Geometry check sheet. Reference: the model listing, model coordinates, mm. Face numbers are marked on the shaded views. Coordinates: 2 decimals unless noted, no trailing zeros. Write each loop counter-clockwise with the first axis right and the second up, starting at its lowest first coordinate (ties: lowest second). Pieces come first, ordered by that corner, then holes. Notation, with made-up numbers: (44, -19) -> (85, -19) arc R21 cw to (85, -11) -> close; hole circle Ø9 at (66.5, 34). An arc over 180 degrees is marked (long way). Answer in a Markdown table with one row per item. Add a question column.
1. Cross-section at B-B on y = -7.5. Record the cut outline in (x, z), and give its area (3 significant figures).
2. Depth check by flat-ended pin: P1, Ø1.5, axis at x = 27.5, y = 3, coming from the +Z side; P2, Ø5, axis at x = 50.5, z = -10.5, coming from the +Y side; P3, Ø4, axis at x = 23, y = 2.5, coming from the +Z side. Enter the tip coordinate at first touch or a pass-through.
3. Cross-section at A-A on x = 14. Record the cut outline in (y, z).
4. Mould release check, pull along Y, two halves, no side actions. Record for the marked faces 1, 2 and 3: pulls with the +Y half, pulls with the -Y half, needs draft (parallel to the pull), parting line crosses it, or undercut.
5. Scan lines: L1, parallel to Z at x = 18, y = -2; L2, parallel to Z at x = 59.5, y = -8.5; L3, parallel to X at y = 13, z = -13.5. Record each from-to range of solid material in increasing order. Write a range as from..to.
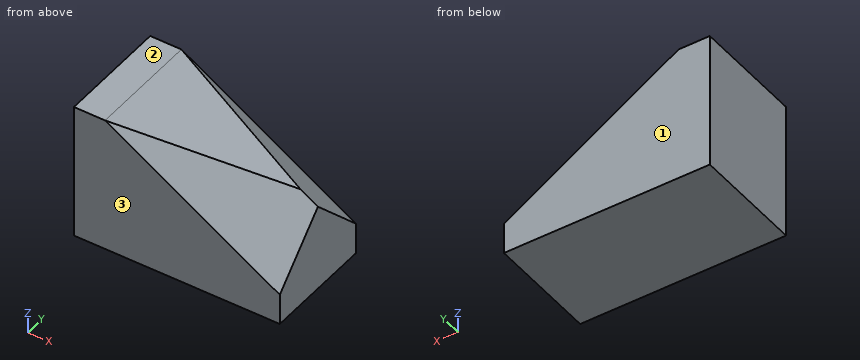
Autodesk Inventor part; units mm, degrees
ref_plane "工作平面1" through (10, 18, 0) normal (-0.3945, -0.6498, -0.6498) x (0.8548, 0, -0.519)
ref_plane "YZ Plane" through (0, 0, 0) normal (1, 0, 0) x (0, 1, 0)
ref_plane "XZ Plane" through (0, 0, 0) normal (0, 1, 0) x (-1, 0, 0)
sketch "草圖1" plane through (0, 0, 0) normal (0, 1, 0) x (-1, 0, 0)
  line L0 (0, 0) -> (-66, 0)
  line L1 (-66, 0) -> (-66, -44)
  line L2 (-66, -44) -> (0, -44)
  line L3 (0, -44) -> (0, 0)
  dimension "d0" = 66
  dimension "d1" = 44
extrude "擠出1" add sketch "草圖1" along normal mid plane 36
sketch "草圖2" plane through (0, 18, 0) normal (0, 1, 0) x (1, 0, 0)
  line L0 (0, 0) -> (66, 0)
  line L1 (10, 0) -> (66, 14)
  line L2 (66, 0) -> (66, 44)
  dimension "d4" = 10
  dimension "d5" = 30
extrude "擠出2" cut sketch "草圖2" against normal blind 40
sketch "草圖3" plane through (66, -18, -44) normal (1, 0, 0) x (0, 0, -1)
  line L0 (-30, 16) -> (-10, 36)
  line L1 (0, 36) -> (-44, 36)
  line L2 (-30, 36) -> (-30, 0)
  point P0 (-44, 18)
  dimension "d8" = 20
  dimension "d9" = 20
ref_plane "工作平面1" through (10, 18, 0) normal (-0.3945, -0.6498, -0.6498) x (0.8548, 0, -0.519)
sketch "草圖4" plane through (10, 18, 0) normal (-0.3945, -0.6498, -0.6498) x (0.8548, 0, -0.519)
  line L0 (-15.1543, -12.3218) -> (93.717, -12.3218)
  line L1 (93.717, -12.3218) -> (93.717, 28.8166)
  line L2 (93.717, 28.8166) -> (-15.1543, 28.8166)
  line L3 (-15.1543, 28.8166) -> (-15.1543, -12.3218)
  point P0 (-8.5479, 10.3104)
extrude "擠出3" cut sketch "草圖4" against normal blind 40
mirror "鏡射1" about plane through (0, 0, 0) normal (0, 1, 0) of "擠出3"
properties part number "25"
Results found:
| question | item | result |
|---|---|---|
| 1 | outline | (0, -44) -> (66, -44) -> (66, -23.5) -> (39.39, -7.35) -> (10, 0) -> (0, 0) -> close |
| 1 | area | 2,390 mm^2 |
| 2 | P1 | stops at z = -4.19 |
| 2 | P2 | stops at y = 6.83 |
| 2 | P3 | stops at z = -2.75 |
| 3 | outline | (-18, -44) -> (18, -44) -> (18, -2.43) -> (16.57, -1) -> (-16.57, -1) -> (-18, -2.43) -> close |
| 4 | face 1 | pulls with the +Y half |
| 4 | face 2 | needs draft |
| 4 | face 3 | pulls with the -Y half |
| 5 | L1 | z = -44..-2 |
| 5 | L2 | z = -44..-20.56 |
| 5 | L3 | x = 0..40.47 |
